```python
from build123d import *

# Parameters (mm, degrees)
SKETCH1_R           = 25
BOSS_EXTRUDE1_DEPTH = 45
BOSS_EXTRUDE2_DEPTH = 35
BOSS_EXTRUDE3_DEPTH = 10
SKETCH2_R           = 16
CUT_EXTRUDE1_DEPTH  = 82
SKETCH3_R           = 10
BOSS_EXTRUDE6_DEPTH = 13
BOSS_EXTRUDE7_START = 3
SKETCH6_R           = 19
SKETCH6_R_2         = 10
BOSS_EXTRUDE7_DEPTH = 3
SKETCH7_R           = 19
SKETCH7_R_2         = 10
BOSS_EXTRUDE8_DEPTH = 3


with BuildPart() as part:
    # Sketch1 → Boss-Extrude1 (new body)
    with BuildSketch(Plane(origin=(0, 0, 0), x_dir=(1, 0, 0), z_dir=(0, 1, 0))):
        with Locations(Location((0, -16, 0), (0, 0, 90))):
            Circle(SKETCH1_R)
    extrude(amount=BOSS_EXTRUDE1_DEPTH)

    # Sketch1_3 → Boss-Extrude2 (add)
    with BuildSketch(Plane(origin=(0, 0, 0), x_dir=(1, 0, 0), z_dir=(0, 1, 0))):
        with BuildLine():
            ThreePointArc((0, 9), (17.67766953, 1.67766953), (25, -16))
            Line((25, -16), (25, 13.01303268))
            Line((25, 13.01303268), (0, 13.01303268))
            Line((0, 13.01303268), (0, 9))
        make_face()
        with BuildLine():
            Line((-25, 13.01303268), (-25, -16))
            ThreePointArc((-25, -16), (-17.67766953, 1.67766953), (0, 9))
            Line((0, 9), (0, 13.01303268))
            Line((0, 13.01303268), (-25, 13.01303268))
        make_face()
        with BuildLine():
            Line((-29.678093712, 13.01303268), (-25, 13.01303268))
            Line((-25, 13.01303268), (0, 13.01303268))
            Line((0, 13.01303268), (0, 23.01303268))
            Line((0, 23.01303268), (-29.678093712, 23.01303268))
            ThreePointArc((-29.678093712, 23.01303268), (-31.799414055, 23.891712336), (-32.678093712, 26.01303268))
            Line((-32.678093712, 26.01303268), (-32.678093712, 44))
            Line((-32.678093712, 44), (-75, 44))
            Line((-75, 44), (-75, 34))
            Line((-75, 34), (-71, 34))
            Line((-71, 34), (-65, 34))
            Line((-65, 34), (-48.678093712, 34))
            ThreePointArc((-48.678093712, 34), (-44.435453024, 32.242640687), (-42.678093712, 28))
            Line((-42.678093712, 28), (-42.678093712, 26.01303268))
            ThreePointArc((-42.678093712, 26.01303268), (-38.870481867, 16.820644525), (-29.678093712, 13.01303268))
        make_face()
        with BuildLine():
            Line((0, 13.01303268), (25, 13.01303268))
            Line((25, 13.01303268), (34.321906288, 13.01303268))
            ThreePointArc((34.321906288, 13.01303268), (43.514294444, 16.820644525), (47.321906288, 26.01303268))
            Line((47.321906288, 26.01303268), (47.321906288, 28))
            ThreePointArc((47.321906288, 28), (49.079265601, 32.242640687), (53.321906288, 34))
            Line((53.321906288, 34), (65, 34))
            Line((65, 34), (71, 34))
            Line((71, 34), (75, 34))
            Line((75, 34), (75, 44))
            Line((75, 44), (37.321906288, 44))
            Line((37.321906288, 44), (37.321906288, 26.01303268))
            ThreePointArc((37.321906288, 26.01303268), (36.443226632, 23.891712336), (34.321906288, 23.01303268))
            Line((34.321906288, 23.01303268), (0, 23.01303268))
            Line((0, 23.01303268), (0, 13.01303268))
        make_face()
    extrude(amount=BOSS_EXTRUDE2_DEPTH)

    # Sketch1_4 → Boss-Extrude3 (add)
    with BuildSketch(Plane(origin=(0, 0, 0), x_dir=(1, 0, 0), z_dir=(0, 1, 0))):
        with BuildLine():
            Line((-45, -16), (-45, -44))
            Line((-45, -44), (0, -44))
            Line((0, -44), (0, -41))
            ThreePointArc((0, -41), (-17.67766953, -33.67766953), (-25, -16))
            Line((-25, -16), (-25, 13.01303268))
            Line((-25, 13.01303268), (-29.678093712, 13.01303268))
            ThreePointArc((-29.678093712, 13.01303268), (-38.870481867, 16.820644525), (-42.678093712, 26.01303268))
            Line((-42.678093712, 26.01303268), (-42.678093712, 28))
            ThreePointArc((-42.678093712, 28), (-44.435453024, 32.242640687), (-48.678093712, 34))
            Line((-48.678093712, 34), (-65, 34))
            Line((-65, 34), (-71, 34))
            ThreePointArc((-71, 34), (-66.757359313, 32.242640687), (-65, 28))
            Line((-65, 28), (-65, 2))
            ThreePointArc((-65, 2), (-63.242640687, -2.242640687), (-59, -4))
            Line((-59, -4), (-57, -4))
            ThreePointArc((-57, -4), (-48.514718626, -7.514718626), (-45, -16))
        make_face()
        with BuildLine():
            Line((0, -41), (0, -44))
            Line((0, -44), (45, -44))
            Line((45, -44), (45, -16))
            ThreePointArc((45, -16), (48.514718626, -7.514718626), (57, -4))
            Line((57, -4), (59, -4))
            ThreePointArc((59, -4), (63.242640687, -2.242640687), (65, 2))
            Line((65, 2), (65, 28))
            ThreePointArc((65, 28), (66.757359313, 32.242640687), (71, 34))
            Line((71, 34), (65, 34))
            Line((65, 34), (53.321906288, 34))
            ThreePointArc((53.321906288, 34), (49.079265601, 32.242640687), (47.321906288, 28))
            Line((47.321906288, 28), (47.321906288, 26.01303268))
            ThreePointArc((47.321906288, 26.01303268), (43.514294444, 16.820644525), (34.321906288, 13.01303268))
            Line((34.321906288, 13.01303268), (25, 13.01303268))
            Line((25, 13.01303268), (25, -16))
            ThreePointArc((25, -16), (17.67766953, -33.67766953), (0, -41))
        make_face()
    extrude(amount=BOSS_EXTRUDE3_DEPTH)

    # Sketch2 → Cut-Extrude1 (cut)
    with BuildSketch(Plane(origin=(0, 45, 0), x_dir=(1, 0, 0), z_dir=(0, 1, 0))):
        with Locations(Location((0, -16, 0), (0, 0, 270))):
            Circle(SKETCH2_R)
    extrude(amount=-CUT_EXTRUDE1_DEPTH, mode=Mode.SUBTRACT)

    # Sketch3 → Boss-Extrude6 (add)
    with BuildSketch(Plane(origin=(45, 0, 0), x_dir=(0, 0, -1), z_dir=(1, 0, 0))):
        with BuildLine():
            Line((17, 0), (-44, 0))
            Line((-44, 0), (-34.771282059, -58.939212458))
            ThreePointArc((-34.771282059, -58.939212458), (-16, -75), (2.771282059, -58.939212458))
            Line((2.771282059, -58.939212458), (17, 0))
        make_face()
        with Locations((-16, -56)):
            Circle(SKETCH3_R, mode=Mode.SUBTRACT)
    boss_extrude6 = extrude(amount=-BOSS_EXTRUDE6_DEPTH)

    # Sketch6 → Boss-Extrude7 (add)
    with BuildSketch(Plane(origin=(45, 0, 0), x_dir=(0, 0, -1), z_dir=(1, 0, 0)).offset(BOSS_EXTRUDE7_START)):
        with Locations((-16, -56)):
            Circle(SKETCH6_R)
        with Locations((-16, -56)):
            Circle(SKETCH6_R_2, mode=Mode.SUBTRACT)
    boss_extrude7 = extrude(amount=-BOSS_EXTRUDE7_DEPTH)

    # Sketch7 → Boss-Extrude8 (add)
    with BuildSketch(Plane.ZY.offset(-32)):
        with Locations(Location((16, -56, 0), (0, 0, 180))):
            Circle(SKETCH7_R)
        with Locations(Location((16, -56, 0), (0, 0, 180))):
            Circle(SKETCH7_R_2, mode=Mode.SUBTRACT)
    boss_extrude8 = extrude(amount=BOSS_EXTRUDE8_DEPTH)

    # Mirror1: Boss-Extrude6, Boss-Extrude7, Boss-Extrude8 across plane
    add(boss_extrude6.mirror(Plane(origin=(0, 0, 0), x_dir=(0, 0, 1), z_dir=(1, 0, 0))))
    add(boss_extrude7.mirror(Plane(origin=(0, 0, 0), x_dir=(0, 0, 1), z_dir=(1, 0, 0))))
    add(boss_extrude8.mirror(Plane(origin=(0, 0, 0), x_dir=(0, 0, 1), z_dir=(1, 0, 0))))


solid = part.part
```
Check sheet for the modelled part. Datum: model origin and axes. Units: mm. A direction names the side the tool comes from. Give positions to 0.01 mm unless a question says otherwise; leave off trailing zeros. Write each loop counter-clockwise with the first axis right and the second up, starting at its lowest first coordinate (ties: lowest second). Pieces come first, ordered by that corner, then holes.
Item 1: Cross-section at B-B (x = 0). Enter the section's corners in (y, z), and give its area (3 significant figures).
Item 2: Access from +Z, -Z, +X, -X, +Y, -Y to the whole of each face (thin tool, end or side, straight path). Record for faces 1 (the face through (-65, 5, -15)), 2 (the face through (48, -64, 8)), 3 (the face through (65, 5, -15)).
Item 3: Cross-section at D-D (z = -19). Enter the section's corners in (x, y).
Item 4: Scan lines: L1, parallel to Y at x = -37, z = 16; L2, parallel to X at y = -52.5, z = 2.5; L3, parallel to X at y = -2, z = 15.5. Record each from-to range of solid material in increasing order.
Item 5: Cross-section at A-A (y = 13). Enter the section's corners in (x, z), and give its area (3 significant figures).
Item 6: Cross-section at C-C (y = -56). Count the separate pieces of the cut face and the enclosed holes in it, and give its area (3 significant figures).
Item 7: Draft check along Y on faces 4 (the face through (38.591, -29.882, -9.786)), 5 (the face through (-38.633, -47.128, 11.386)), 6 (the face through (-62, 21, -34)). Enter one of: released by +Y, released by -Y, zero draft, split by the parting line, or undercut.
Item 8: Gauge pin test, flat ends, axial feed: pin 1 (11.5 mm diameter, centred on y = -64.5, z = 18.5, fed in from +X); pin 2 (1.5 mm diameter, centred on x = 44, y = -15.5, fed in from -Z); pin 3 (19 mm diameter, centred on y = -55, z = 25, fed in from -X); pin 4 (18 mm diameter, centred on y = -56, z = 16, fed in from +X). Record the tip position at first contact, or that the pin passes through.
Report:
1. outline: (0, -23.01) - (35, -23.01) - (35, -9) - (45, -9) - (45, 0) - (0, 0) - close; (0, 32) - (45, 32) - (45, 41) - (10, 41) - (10, 44) - (0, 44) - close
1. area: 1,330 mm2
2. face 1: +Z, -X, +Y, -Y
2. face 2: +Z, -Z, +X, -Y
2. face 3: +Z, +X, +Y, -Y
3. outline: (-65, 0) - (65, 0) - (65, 10) - (45.27, 10) - (45.27, 35) - (-40.62, 35) - (-40.62, 10) - (-65, 10) - close
4. L1: y = -75 to -66, -46 to 10
4. L2: x = -48 to -29, 29 to 48
4. L3: x = -45 to -32, 32 to 45
5. outline: (-75, -44) - (-32.68, -44) - (-32.68, -26.01) arc R3 cw to (-29.68, -23.01) - (34.32, -23.01) arc R3 cw to (37.32, -26.01) - (37.32, -44) - (75, -44) - (75, -34) - (53.32, -34) arc R6 cw to (47.32, -28) - (47.32, -26.01) arc R13 ccw to (34.32, -13.01) - (25, -13.01) - (25, 16) arc R25 ccw to (-25, 16) - (-25, -13.01) - (-29.68, -13.01) arc R13 ccw to (-42.68, -26.01) - (-42.68, -28) arc R6 cw to (-48.68, -34) - (-75, -34) - close; hole circle Ø32 at (0, 16)
5. area: 3,490 mm2
6. separate pieces: 4
6. enclosed holes: 0
6. area: 703 mm2
7. face 4: released by -Y
7. face 5: undercut
7. face 6: zero draft
8. pin 1: stops at x = 48
8. pin 2: stops at z = -13.44
8. pin 3: stops at x = -48
8. pin 4: passes through
